from build123d import *

# Parameters (mm, degrees)
SKETCH1_W           = 38.1
SKETCH1_H           = 25.4
BOSS_EXTRUDE1_DEPTH = 17.018
SKETCH4_W           = 38.1
SKETCH4_H           = 23.368
SKETCH4_R           = 2.794
BOSS_EXTRUDE2_DEPTH = 2.54
CUT_EXTRUDE1_DEPTH  = 62.055704041
BOSS_EXTRUDE3_DEPTH = 22.86
BOSS_EXTRUDE5_DEPTH = 30.734
SKETCH11_R          = 2.0193
CUT_EXTRUDE3_DEPTH  = 30.734
BOSS_EXTRUDE4_DEPTH = 30.734


with BuildPart() as part:
    # Sketch1 → Boss-Extrude1 (new body)
    with BuildSketch(Plane.XY):
        with Locations((19.05, 12.7)):
            Rectangle(SKETCH1_W, SKETCH1_H)
    extrude(amount=BOSS_EXTRUDE1_DEPTH)

    # Sketch4 → Boss-Extrude2 (add)
    with BuildSketch(Plane(origin=(0, 25.4, 0), x_dir=(1, 0, 0), z_dir=(0, 1, 0))):
        with Locations((19.05, -28.702)):
            Rectangle(SKETCH4_W, SKETCH4_H)
        with Locations(Location((6.35, -32.724779192, 0), (0, 0, 270))):
            Circle(SKETCH4_R, mode=Mode.SUBTRACT)
        with Locations(Location((31.75, -30.725755838, 0), (0, 0, 270))):
            Circle(SKETCH4_R, mode=Mode.SUBTRACT)
    extrude(amount=-BOSS_EXTRUDE2_DEPTH)

    # Sketch5 → Cut-Extrude1 (cut, through all)
    with BuildSketch(Plane(origin=(0, 25.4, 0), x_dir=(1, 0, 0), z_dir=(0, 1, 0))):
        Polygon((38.1, -36.576), (0, -39.57453503), (0, -40.386), (38.1, -40.386), align=None)
    extrude(amount=-CUT_EXTRUDE1_DEPTH, mode=Mode.SUBTRACT)

    # Sketch7 → Boss-Extrude3 (add)
    with BuildSketch(Plane.XZ):
        Polygon((38.1, 17.018), (0, 20.01653503), (0, 17.018), align=None)
    extrude(amount=-BOSS_EXTRUDE3_DEPTH)

    # Sketch10 → Boss-Extrude5 (add)
    with BuildSketch(Plane.XZ):
        Polygon((0, 0), (0, 20.01653503), (38.1, 17.018), (38.1, 0), align=None)
    extrude(amount=BOSS_EXTRUDE5_DEPTH)

    # Sketch11 → Cut-Extrude3 (cut)
    with BuildSketch(Plane(origin=(0, 0, 0), x_dir=(-1, 0, 0), z_dir=(0, 0, -1))):
        with Locations((-25.4, -2.794)):
            Circle(SKETCH11_R)
        with Locations((-12.7, -2.794)):
            Circle(SKETCH11_R)
    extrude(amount=-CUT_EXTRUDE3_DEPTH, mode=Mode.SUBTRACT)

    # Sketch9 → Boss-Extrude4 (add)
    with BuildSketch(Plane.XZ):
        Polygon((0, 0), (38.1, 0), (38.1, 17.018), (0, 20.01653503), align=None)
    extrude(amount=BOSS_EXTRUDE4_DEPTH)


solid = part.part
Input: part model. Units: mm. Frame: model coordinates. A direction names the side the tool comes from. Coordinates: 2 decimals unless noted, no trailing zeros. Order: outer loops, then holes, each group sorted by start corner. A loop starts at its lowest first (then second) coordinate and runs counter-clockwise, first axis right, second up. Notation, with made-up numbers: M 20,74.5 L 50,74.5 A24 ccw 50,110.5 Z; hole C 56,20 d11. An arc over 180 degrees is marked long. Write item = value, one per line. Start each with the question number.
(1) Section C-C on x = 19.5. Output: boundary loops of the cut face in (y, z).
(2) Section A-A on x = 31.75. Output: boundary loops of the cut face in (y, z).
(3) Reachability of faces 1 (the flat face through (18.78, -3.56, 18.54)), 2 (the flat face through (19, -2, 0)) from +Z, -Z, +X, -X, +Y, -Y: full face, straight path, thin tool, end or side. Return the list, or none.
(4) First-contact query: P1, Ø3, axis at x = 23.5, y = 19.5, coming from the +Z side; P2, Ø3, axis at x = 30.5, y = -20.5, coming from the +Z side; P3, Ø7, axis at x = 15, z = 27, coming from the -Y side. Flat tips, straight axial feed; report the tip coordinate or a pass-through.
(5) Section B-B on y = -25. Output: boundary loops of the cut face in (x, z).
(6) Section D-D on z = 22.5. Output: boundary loops of the cut face in (x, y), and give its area (3 significant figures).
(7) Line query: line 1 along Y through (x, z) = (34.5, 25); line 2 along Z through (x, y) = (6, 23); line 3 along Z through (x, y) = (31, 24). Output: solid intervals per line, ascending. Write a range as [from, to].
Result set:
q1.outline = M -30.73,0 L 25.4,0 L 25.4,38.04 L 22.86,38.04 L 22.86,18.48 L -30.73,18.48 Z
q2.outline = M -30.73,0 L 25.4,0 L 25.4,27.93 L 22.86,27.93 L 22.86,17.52 L -30.73,17.52 Z; M 22.86,33.52 L 25.4,33.52 L 25.4,37.08 L 22.86,37.08 Z
q3.face_1 = +Z, +X, -Y
q3.face_2 = -Z, +X, -X, +Y, -Y
q4.P1 = 18.29
q4.P2 = 17.73
q4.P3 = 22.86
q5.outline = M 0,0 L 38.1,0 L 38.1,17.02 L 0,20.02 Z
q6.outline = M 0,22.86 L 38.1,22.86 L 38.1,25.4 L 0,25.4 Z
q6.area = 96.8 mm²
q7.line_1 = [22.86, 25.4]
q7.line_2 = [0, 29.95], [35.5, 39.1]
q7.line_3 = [0, 28.03], [33.42, 37.13]
